Geometry: see drawing. Coordinates: mm, zero at the bounding-box minimum. Round coordinates to 2 decimals unless told otherwise and drop trailing zeros. Loops run counter-clockwise (first coordinate to the right, second up) from the corner with the lowest first, then second, coordinate; pieces in that order, holes last. Notation, with made-up numbers: M 47.25,-12.75 L 103.25,-12.75 A21 cw 103.25,-7.75 Z; hole C 55.25,87.5 d11. An arc over 180 degrees is marked long. Answer as a JSON object with one key per item and string values.
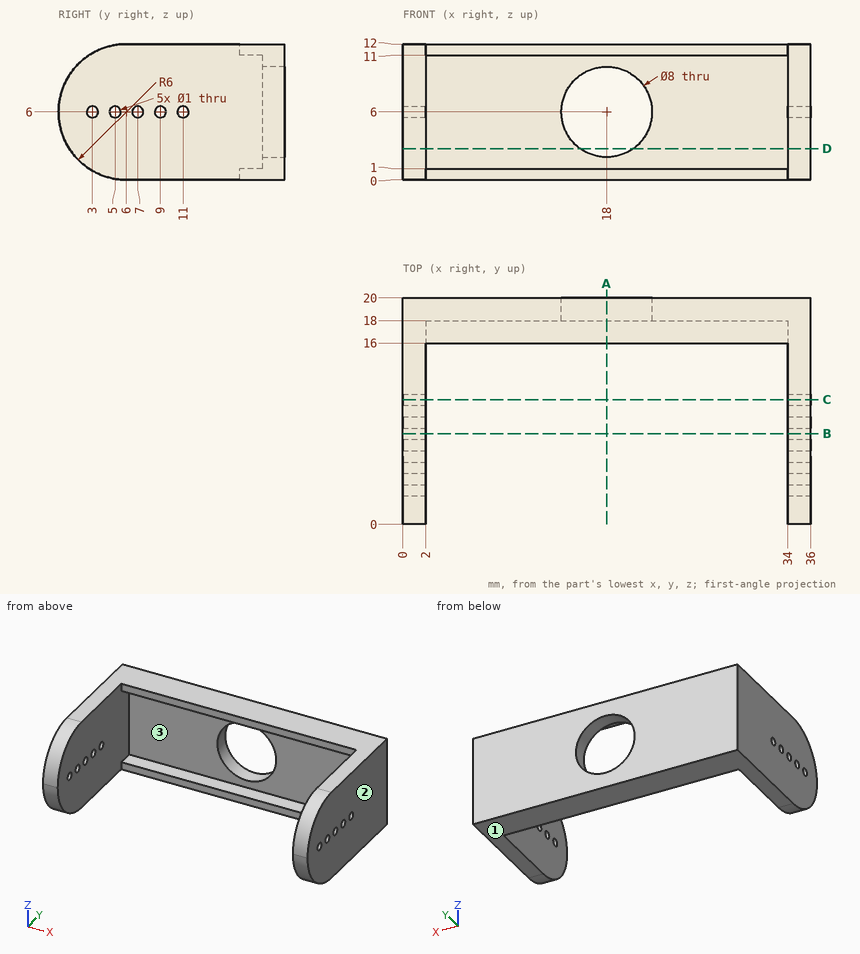
1) Section query C-C (y = 11). Return the cut outline in (x, z).
Results:
{"outline": "M 0,0 L 2,0 L 2,5.5 L 0,5.5 Z; M 0,6.5 L 2,6.5 L 2,12 L 0,12 Z; M 34,0 L 36,0 L 36,5.5 L 34,5.5 Z; M 34,6.5 L 36,6.5 L 36,12 L 34,12 Z"}
2) Ray query, line 1 (X direction, y = 8.75, z = 1.5); line 2 (X direction, y = 18.6, z = 6); line 3 (Y direction, x = 16.5, z = 1.25). Return the intervals inside material, ascending.
Results:
{"line 1": "0 to 2, 34 to 36", "line 2": "0 to 14, 22 to 36", "line 3": "18 to 20"}
3) Section query D-D (z = 2.75). Return the cut outline in (x, y).
Results:
{"outline": "M 0,0.96 L 2,0.96 L 2,18 L 15.67,18 L 15.67,20 L 0,20 Z; M 20.33,18 L 34,18 L 34,0.96 L 36,0.96 L 36,20 L 20.33,20 Z"}
4) Section query A-A (x = 18). Return the cut outline in (y, z), and give its area (3 significant figures).
Results:
{"outline": "M 16,0 L 20,0 L 20,2 L 18,2 L 18,1 L 16,1 Z; M 16,11 L 18,11 L 18,10 L 20,10 L 20,12 L 16,12 Z", "area": "12.0 mm2"}
5) Pull-direction query (Z, two-part tool) for the marked faces 1, 2 and 3; classes: +Z half, -Z half, draft (parallel to the pull), parting line (faces both ways), or undercut.
Results:
{"face 1": "-Z half", "face 2": "draft", "face 3": "undercut"}
6) Section query B-B (y = 8). Return the cut outline in (x, z).
Results:
{"outline": "M 0,0 L 2,0 L 2,12 L 0,12 Z; M 34,0 L 36,0 L 36,12 L 34,12 Z"}
7) Pin query (flat end, axial travel): P1, Ø1.1, axis at x = 22, z = 11.5, coming from the -Y side; P2, Ø6, axis at y = 5, z = 6.5, coming from the -X side; P3, Ø10, axis at x = 9, y = 7, coming from the -Z side. Return the tip coordinate at first contact, or that it passes through.
Results:
{"P1": "y = 16", "P2": "x = 0", "P3": "through"}
